```python
from build123d import *

# Parameters (mm, degrees)
F0_W           = 53.960219
F0_H           = 33.172701
F1_DEPTH       = 25.4
F2_R           = 3.81
F3_R           = 6.35
F4_DEPTH       = 25.401
F6_D           = 6.35
F6_CBORE_D     = 12.7
F6_CBORE_DEPTH = 6.35


with BuildPart() as f1:
    # F0 (on Front) → F1 (new body)
    with BuildSketch(Plane.XZ):
        with Locations((26.980109, 16.58635)):
            Rectangle(F0_W, F0_H)
    extrude(amount=F1_DEPTH)

    # F2
    f2_edges = [f1.edges().sort_by_distance(p)[0] for p in [
        (26.98011, -25.4, 33.172701),
        (53.960219, -12.7, 33.172701),
        (0, -25.4, 16.58635),
        (26.98011, -25.4, 0),
        (53.960219, -25.4, 16.58635),
        (53.960219, -12.7, 0),
        (53.960219, 0, 16.58635),
        (0, 0, 16.58635),
        (26.98011, 0, 0),
        (26.98011, 0, 33.172701),
        (0, -12.7, 33.172701),
        (0, -12.7, 0),
    ]]
    fillet(f2_edges, radius=F2_R)

    # F3 (on face) → F4 (cut, through all)
    with BuildSketch(Plane.XZ.offset(25.4)):
        with Locations((27.24513, 17.117795)):
            Circle(F3_R)
    extrude(amount=-F4_DEPTH, mode=Mode.SUBTRACT)

    # F6 (through all)
    with Locations(Plane.XY.offset(33.172701)):
        with Locations((12.7, -12.7), (41.260219, -12.7)):
            CounterBoreHole(F6_D / 2, F6_CBORE_D / 2, F6_CBORE_DEPTH)


solid = f1.part
```
Check sheet for the modelled part. Datum: model origin and axes. Units: mm. A direction names the side the tool comes from. Coordinates: 2 decimals unless noted, no trailing zeros. Write each loop counter-clockwise with the first axis right and the second up, starting at its lowest first coordinate (ties: lowest second). Pieces come first, ordered by that corner, then holes. Notation, with made-up numbers: (53, -7) -> (63, -7) arc R8 cw to (63, 3) -> close; hole circle Ø2 at (-1, 86.5). An arc over 180 degrees is marked (long way). Use a Markdown table: item, result.
1. Go/stop test with flat-tipped pins: pin 1 Ø10 at (x, y) = (41.26, -12.7) entering from +Z; pin 2 Ø10 at (x, z) = (27.25, 17.12) entering from -Y. Record where each tip stops, or that it passes through.
Reported:
| item | result |
|---|---|
| pin 1 | stops at z = 26.82 |
| pin 2 | passes through |
2. Sectioned sample at D-D (x = 12.7). Enter the section's corners in (y, z) (3 decimals).
Reported:
| item | result |
|---|---|
| outline | (-25.4, 3.81) arc R3.81 ccw to (-21.59, 0) -> (-15.875, 0) -> (-15.875, 26.823) -> (-19.05, 26.823) -> (-19.05, 33.173) -> (-21.59, 33.173) arc R3.81 ccw to (-25.4, 29.363) -> close; (-9.525, 0) -> (-3.81, 0) arc R3.81 ccw to (0, 3.81) -> (0, 29.363) arc R3.81 ccw to (-3.81, 33.173) -> (-6.35, 33.173) -> (-6.35, 26.823) -> (-9.525, 26.823) -> close |
3. Sectioned sample at C-C (y = -12.7). Enter the section's corners in (x, z) (3 decimals), plus the area to 3 significant figures.
Reported:
| item | result |
|---|---|
| outline | (0, 3.81) arc R3.81 ccw to (3.81, 0) -> (9.525, 0) -> (9.525, 26.823) -> (6.35, 26.823) -> (6.35, 33.173) -> (3.81, 33.173) arc R3.81 ccw to (0, 29.363) -> close; (15.875, 0) -> (38.085, 0) -> (38.085, 26.823) -> (34.91, 26.823) -> (34.91, 33.173) -> (19.05, 33.173) -> (19.05, 26.823) -> (15.875, 26.823) -> close; (44.435, 0) -> (50.15, 0) arc R3.81 ccw to (53.96, 3.81) -> (53.96, 29.363) arc R3.81 ccw to (50.15, 33.173) -> (47.61, 33.173) -> (47.61, 26.823) -> (44.435, 26.823) -> close; hole circle Ø12.7 at (27.245, 17.118) |
| area | 1,150 mm2 |
4. Release check for a two-part mould opening along Z. For faces 3 (the cylindrical face through (27.304, -24.254, 1.086)), 4 (the cylindrical face through (1.086, -1.146, 16.765)), 5 (the cylindrical face through (22.565, -12.878, 21.409)) record: pulls with the +Z half, pulls with the -Z half, needs draft (parallel to the pull), parting line crosses it, or undercut.
Reported:
| item | result |
|---|---|
| face 3 | pulls with the -Z half |
| face 4 | needs draft |
| face 5 | undercut |
5. Sectioned sample at B-B (z = 16). Enter the section's corners in (x, y) (3 decimals).
Reported:
| item | result |
|---|---|
| outline | (0, -21.59) arc R3.81 ccw to (3.81, -25.4) -> (20.994, -25.4) -> (20.994, 0) -> (3.81, 0) arc R3.81 ccw to (0, -3.81) -> close; (33.496, -25.4) -> (50.15, -25.4) arc R3.81 ccw to (53.96, -21.59) -> (53.96, -3.81) arc R3.81 ccw to (50.15, 0) -> (33.496, 0) -> close; hole circle Ø6.35 at (12.7, -12.7); hole circle Ø6.35 at (41.26, -12.7) |
6. Sectioned sample at A-A (z = 27.5). Enter the section's corners in (x, y).
Reported:
| item | result |
|---|---|
| outline | (0, -21.59) arc R3.81 ccw to (3.81, -25.4) -> (50.15, -25.4) arc R3.81 ccw to (53.96, -21.59) -> (53.96, -3.81) arc R3.81 ccw to (50.15, 0) -> (3.81, 0) arc R3.81 ccw to (0, -3.81) -> close; hole circle Ø12.7 at (12.7, -12.7); hole circle Ø12.7 at (41.26, -12.7) |
7. Tool access check on faces 1 (the flat face through (15.4, -15.4, 26.823)), 2 (the cylindrical face through (11.2, -15.5, 13.2)). Record the directions out of +Z, -Z, +X, -X, +Y, -Y that give a thin tool (end or side, any length) a straight path to the whole face; none if there is none.
Reported:
| item | result |
|---|---|
| face 1 | +Z |
| face 2 | +Z, -Z |
8. Scan lines: line 1 along Y through (x, z) = (13, 25.5); line 2 along X through (y, z) = (-2, 23); line 3 along Z through (x, y) = (45.5, -11.5). Record each from-to range of solid material in increasing order.
Reported:
| item | result |
|---|---|
| line 1 | y = -25.4 to -15.86, -9.54 to 0 |
| line 2 | x = 0.46 to 24.85, 29.64 to 53.5 |
| line 3 | z = 0 to 26.82 |
